Read the model definition and answer for the solid it produces. Units are mm, in the model's axes. Face numbers are marked on the shaded views. A direction names the side the tool comes from. Give positions to 0.01 mm unless a question says otherwise; leave off trailing zeros. Order: outer loops, then holes, each group sorted by start corner. A loop starts at its lowest first (then second) coordinate and runs counter-clockwise, first axis right, second up. Notation, with made-up numbers: (46.25, 1.5) - (59.25, 1.5) arc R31 cw to (59.25, 38.5) - close; hole circle Ø5 at (-9.75, 63.5). An arc over 180 degrees is marked (long way). Use a Markdown table: item, result. Add a question column.
1. A cutting plane is placed at B-B on z = 0. Determine the outline of the cut face in (x, y).
2. For a pull along Z with two mould halves and no side action, classify the marked faces 3, 4, 5 and 6 as released by +Z, released by -Z, zero draft, split by the parting line, or undercut.
3. A cutting plane is placed at A-A on y = -32.5. Determine the outline of the cut face in (x, z), and give its area (3 significant figures).
4. Which of the six approach directions +Z, -Z, +X, -X, +Y, -Y give full straight-line access (tool end or side, diameter ignored) to the marked faces 1 and 2?
5. A cutting plane is placed at C-C on z = -72. Determine the outline of the cut face in (x, y).
6. Flat-ended cylindrical pins translate along their axes: P1, Ø1, axis at x = 7.5, y = -0.5, coming from the -Z side; P2, Ø12, axis at x = 90, z = -15, coming from the +Y side; P3, Ø1.4, axis at x = 5.5, y = -0.5, coming from the +Z side. Find the tip coordinate at first contact, or state that the pin passes through.
7. Consider L1, parallel to Z at x = 165, y = -27.5; L2, parallel to X at y = -29, z = 14; L3, parallel to Y at x = 40, z = 44. Determine where each line is inside the solid, lowest interval first.
8. A cutting plane is placed at D-D on x = 109. Determine the outline of the cut face in (y, z), and give its area (3 significant figures).
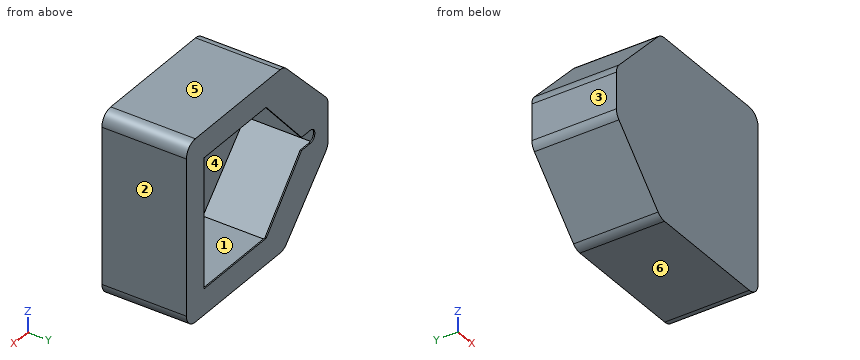
```python
from build123d import *

# Parameters (mm, degrees)
F1_DEPTH = 1.27
F3_DEPTH = 76.2
F5_DEPTH = 5.08
F6_R     = 12.7
F7_R     = 12.7


with BuildPart() as f1:
    # F0 (on Front) → F1 (new body)
    with BuildSketch(Plane.XZ):
        Polygon((-25.4, 22.8833369911), (-25.4, 0), (-25.4, -22.8833369911), (38.1, -88.9), (177.8, -88.9), (177.8, 0), (177.8, 88.9), (38.1, 88.9), align=None)
        with BuildLine():
            Line((0, 6.35), (12.7, 6.35))
            Line((12.7, 6.35), (63.5, 63.5))
            Line((63.5, 63.5), (152.4, 63.5))
            Line((152.4, 63.5), (152.4, 0))
            Line((152.4, 0), (152.4, -63.5))
            Line((152.4, -63.5), (63.5, -63.5))
            Line((63.5, -63.5), (12.7, -6.35))
            Line((12.7, -6.35), (0, -6.35))
            ThreePointArc((0, -6.35), (-6.35, 0), (0, 6.35))
        make_face(mode=Mode.SUBTRACT)
    extrude(amount=F1_DEPTH)

    # F2 (on face) → F3 (join)
    with BuildSketch(Plane.XZ.offset(1.27)):
        Polygon((38.1, 88.9), (-25.4, 22.8833369911), (-25.4, -22.8833369911), (38.1, -88.9), (177.8, -88.9), (177.8, 88.9), align=None)
        Polygon((40.2622562786, -83.82), (-20.32, -20.8367181565), (-20.32, 20.8367181565), (40.2622562786, 83.82), (172.72, 83.82), (172.72, -83.82), align=None, mode=Mode.SUBTRACT)
    extrude(amount=F3_DEPTH)

    # F4 (on face) → F5 (join)
    with BuildSketch(Plane.XZ.offset(77.47)):
        Polygon((177.8, 88.9), (38.1, 88.9), (-25.4, 22.8833369911), (-25.4, -22.8833369911), (38.1, -88.9), (177.8, -88.9), align=None)
        Polygon((172.72, -83.82), (40.2622562786, -83.82), (-20.32, -20.8367181565), (-20.32, 20.8367181565), (40.2622562786, 83.82), (172.72, 83.82), align=None, mode=Mode.SUBTRACT)
        Polygon((-20.32, -20.8367181565), (40.2622562786, -83.82), (172.72, -83.82), (172.72, 83.82), (40.2622562786, 83.82), (-20.32, 20.8367181565), align=None)
    extrude(amount=F5_DEPTH)

    # F6
    f6_edges = [f1.edges().sort_by_distance(p)[0] for p in [
        (-25.4, -41.275, 22.883337),
        (-25.4, -41.275, -22.883337),
        (38.1, -41.275, 88.9),
        (38.1, -41.275, -88.9),
    ]]
    fillet(f6_edges, radius=F6_R)

    # F7
    f7_edges = [f1.edges().sort_by_distance(p)[0] for p in [
        (177.8, -41.275, 88.9),
        (177.8, -41.275, -88.9),
    ]]
    fillet(f7_edges, radius=F7_R)


solid = f1.part
```
Output values:
| question | item | result |
|---|---|---|
| 1 | outline | (-25.4, -82.55) - (177.8, -82.55) - (177.8, 0) - (152.4, 0) - (152.4, -1.27) - (172.72, -1.27) - (172.72, -77.47) - (-20.32, -77.47) - (-20.32, -1.27) - (-6.35, -1.27) - (-6.35, 0) - (-25.4, 0) - close |
| 2 | face 3 | zero draft |
| 2 | face 4 | undercut |
| 2 | face 5 | released by +Z |
| 2 | face 6 | released by -Z |
| 3 | outline | (-25.4, -17.77) arc R12.7 ccw to (-21.85, -26.57) - (34.35, -85) arc R12.7 ccw to (43.51, -88.9) - (165.1, -88.9) arc R12.7 ccw to (177.8, -76.2) - (177.8, 76.2) arc R12.7 ccw to (165.1, 88.9) - (43.51, 88.9) arc R12.7 ccw to (34.35, 85) - (-21.85, 26.57) arc R12.7 ccw to (-25.4, 17.77) - close; hole (-20.32, -20.84) - (40.26, -83.82) - (172.72, -83.82) - (172.72, 83.82) - (40.26, 83.82) - (-20.32, 20.84) - close |
| 3 | area | 3,310 mm² |
| 4 | face 1 | none |
| 4 | face 2 | +Z, -Z, +X, +Y, -Y |
| 5 | outline | (21.84, -82.55) - (177.8, -82.55) - (177.8, 0) - (21.84, 0) - close; hole (28.89, -77.47) - (172.72, -77.47) - (172.72, -1.27) - (28.89, -1.27) - close |
| 6 | P1 | z = -57.61 |
| 6 | P2 | y = -77.47 |
| 6 | P3 | z = 55.74 |
| 7 | L1 | -88.9 to -83.82, 83.82 to 88.9 |
| 7 | L2 | -25.4 to -20.32, 172.72 to 177.8 |
| 7 | L3 | -82.55 to -77.47, -1.27 to 0 |
| 8 | outline | (-82.55, -88.9) - (0, -88.9) - (0, -63.5) - (-1.27, -63.5) - (-1.27, -83.82) - (-77.47, -83.82) - (-77.47, 83.82) - (-1.27, 83.82) - (-1.27, 63.5) - (0, 63.5) - (0, 88.9) - (-82.55, 88.9) - close |
| 8 | area | 1,740 mm² |
